The listing builds one solid part. Answer for the finished solid, in the listing's coordinates (mm). Coordinates: 2 decimals unless noted, no trailing zeros. Order: outer loops, then holes, each group sorted by start corner. A loop starts at its lowest first (then second) coordinate and runs counter-clockwise, first axis right, second up. Notation, with made-up numbers: (48, -7) -> (95, -7) arc R18 ccw to (95, 18) -> close; hole circle Ø1 at (71.5, 10.5). An arc over 180 degrees is marked (long way). Answer in a Markdown table with one row per item.
```python
from build123d import *

# Parameters (mm, degrees)
SKETCH_1_R      = 4.725
SKETCH_1_R_2    = 1.55
EXTRUDE_1_DEPTH = 42.5
EXTRUDE_START   = -42.5
SKETCH_2_R      = 4.85
SKETCH_2_R_2    = 4.725
EXTRUDE_2_DEPTH = 42.5
SKETCH_3_R      = 4.875
SKETCH_3_R_2    = 4.85
EXTRUDE_3_DEPTH = 42.5
SKETCH_4_R      = 4.95
SKETCH_4_R_2    = 4.875
EXTRUDE_4_DEPTH = 42.5


with BuildPart() as part:
    # 草图1 → 凸台-拉伸1 (new body)
    with BuildSketch(Plane(origin=(0, 0, 0), x_dir=(1, 0, 0), z_dir=(0, 1, 0))):
        with Locations(Location((0, 0, 0), (0, 0, 270))):
            Circle(SKETCH_1_R)
        with Locations(Location((0, 0, 0), (0, 0, 270))):
            Circle(SKETCH_1_R_2, mode=Mode.SUBTRACT)
    extrude(amount=EXTRUDE_1_DEPTH)

    # 草图2 → 凸台-拉伸2 (add)
    with BuildSketch(Plane(origin=(0, 42.5, 0), x_dir=(1, 0, 0), z_dir=(0, 1, 0)).offset(EXTRUDE_START)):
        with Locations(Location((0, 0, 0), (0, 0, 270))):
            Circle(SKETCH_2_R)
        Circle(SKETCH_2_R_2, mode=Mode.SUBTRACT)
    extrude(amount=EXTRUDE_2_DEPTH)

    # 草图3 → 凸台-拉伸3 (add)
    with BuildSketch(Plane.XZ):
        with Locations(Location((0, 0, 0), (0, 0, 270))):
            Circle(SKETCH_3_R)
        Circle(SKETCH_3_R_2, mode=Mode.SUBTRACT)
    extrude(amount=-EXTRUDE_3_DEPTH)

    # 草图4 → 凸台-拉伸4 (add)
    with BuildSketch(Plane.XZ):
        with Locations(Location((0, 0, 0), (0, 0, 270))):
            Circle(SKETCH_4_R)
        Circle(SKETCH_4_R_2, mode=Mode.SUBTRACT)
    extrude(amount=-EXTRUDE_4_DEPTH)


solid = part.part
```
(1) A cutting plane is placed at C-C, the plane y = 11. Determine the outline of the cut face in (x, z), then the cut area to 3 significant figures.
Check values:
| item | result |
|---|---|
| outline | circle Ø9.9 at (0, 0); hole circle Ø3.1 at (0, 0) |
| area | 69.4 mm² |
(2) A cutting plane is placed at D-D, the plane x = 4. Determine the outline of the cut face in (y, z), then the cut area to 3 significant figures.
Check values:
| item | result |
|---|---|
| outline | (0, -2.92) -> (42.5, -2.92) -> (42.5, 2.92) -> (0, 2.92) -> close |
| area | 248 mm² |
(3) For a pull along Z with two mould halves and no side action, classify faces 1 (the cylindrical face through (1.49, 20.95, -4.72)), 2 (the flat face through (-2, 42.5, 0)), 3 (the cylindrical face through (0.466, 20.952, 1.478)) as released by +Z, released by -Z, zero draft, split by the parting line, or undercut.
Check values:
| item | result |
|---|---|
| face 1 | split by the parting line |
| face 2 | zero draft |
| face 3 | undercut |
(4) Find the intervals of material crossed by line 1 along X through (y, z) = (26.5, 0); line 2 along Z through (x, y) = (-0.75, 37); line 3 along Z through (x, y) = (0.25, 16.5), in increasing order. Write a range as from..to.
Check values:
| item | result |
|---|---|
| line 1 | -4.95..-1.55, 1.55..4.95 |
| line 2 | -4.89..-1.36, 1.36..4.89 |
| line 3 | -4.94..-1.53, 1.53..4.94 |
(5) A cutting plane is placed at A-A, the plane x = 0. Determine the outline of the cut face in (y, z), then the cut area to 3 significant figures.
Check values:
| item | result |
|---|---|
| outline | (0, -4.95) -> (42.5, -4.95) -> (42.5, -1.55) -> (0, -1.55) -> close; (0, 1.55) -> (42.5, 1.55) -> (42.5, 4.95) -> (0, 4.95) -> close |
| area | 289 mm² |
(6) A flat-ended cylindrical pin translates along its axis: pin 1 (5 mm diameter, centred on x = -0.5, y = 34.5, fed in from -Z). Find the tip coordinate at first contact, or state that the pin passes through.
Check values:
| item | result |
|---|---|
| pin 1 | z = -4.95 |
(7) A cutting plane is placed at B-B, the plane z = 0. Determine the outline of the cut face in (x, y).
Check values:
| item | result |
|---|---|
| outline | (-4.95, 0) -> (-1.55, 0) -> (-1.55, 42.5) -> (-4.95, 42.5) -> close; (1.55, 0) -> (4.95, 0) -> (4.95, 42.5) -> (1.55, 42.5) -> close |
